The listing builds one solid part. Answer for the finished solid, in the listing's coordinates (mm). Face numbers are marked on the shaded views. A direction names the side the tool comes from. Round coordinates to 2 decimals unless told otherwise and drop trailing zeros. Order: outer loops, then holes, each group sorted by start corner. A loop starts at its lowest first (then second) coordinate and runs counter-clockwise, first axis right, second up. Notation, with made-up numbers: M 63.25,15.5 L 85.25,15.5 A14 ccw 85.25,38.5 Z; hole C 0,59 d4. An arc over 180 degrees is marked long. Put each result on its own line as item: value. Start each with the question number.
1. The mould has two halves that part along X. Classify the marked faces 4 and 5: +X half, -X half, draft (parallel to the pull), parting line (faces both ways), or undercut.
2. The part is cut by section C-C (y = 31.25). Give the vertices of the cut face in (x, z).
3. Which of the six approach directions +Z, -Z, +X, -X, +Y, -Y give full straight-line access (tool end or side, diameter ignored) to the marked faces 1, 2 and 3?
4. The part is cut by section D-D (z = -28.5). Give the vertices of the cut face in (x, y).
5. Each of these flat-tipped pins is pushed along its axis until it touches: pin 1 Ø6 at (x, z) = (58, -15) entering from +Y; pin 2 Ø7 at (x, z) = (15, -16) entering from -Y; pin 3 Ø2 at (y, z) = (30.5, -10.5) entering from -X; pin 4 Ø6.5 at (x, z) = (60, -16) entering from -Y. Where does it stop, or does it pass through?
6. The part is cut by section A-A (y = 23.75). Give the vertices of the cut face in (x, z).
7. Consider line 1 (X direction, y = 32.5, z = -16); line 2 (Z direction, x = 60, y = 25.75); line 3 (X direction, y = 23.75, z = -16). Determine where each line is inside the solid, lowest interval first.
8. The part is cut by section B-B (x = -60). Give the vertices of the cut face in (y, z).
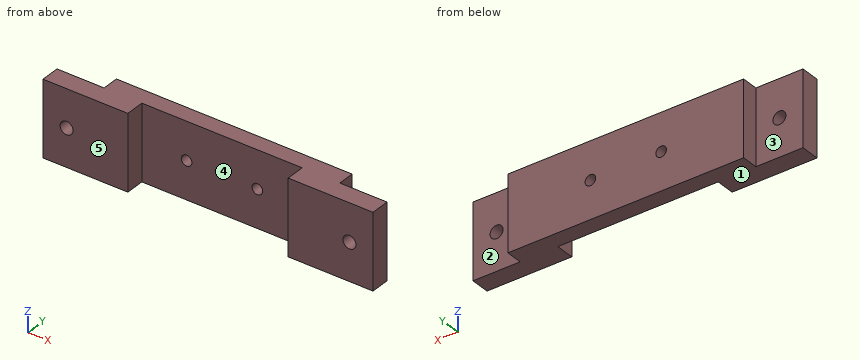
from build123d import *

# Parameters (mm, degrees)
AUFSATZ_LINEAR_AUSTRAGEN1_DEPTH  = 32
F_4_5_4_5_DURCHMESSER_BOHRUNG1_D = 4.5
F_5_5_5_5_DURCHMESSER_BOHRUNG1_D = 5.5


with BuildPart() as part:
    # Skizze1 → Aufsatz-Linear austragen1 (new body)
    with BuildSketch(Plane.XY):
        Polygon((-70, 20), (-34, 20), (-34, 28), (34, 28), (34, 20), (70, 20), (70, 28), (50, 28), (50, 35), (-50, 35), (-50, 28), (-70, 28), align=None)
    extrude(amount=-AUFSATZ_LINEAR_AUSTRAGEN1_DEPTH)

    # Ø4.5 (4.5) Durchmesser Bohrung1 (through all)
    with Locations(Plane(origin=(-15, 28, -16), x_dir=(0, 0, -1), z_dir=(0, -1, 0))):
        with Locations((0, 0), (0, 30)):
            Hole(F_4_5_4_5_DURCHMESSER_BOHRUNG1_D / 2)

    # Ø5.5 (5.5) Durchmesser Bohrung1 (through all)
    with Locations(Plane(origin=(-60, 28, -16), x_dir=(1, 0, 0), z_dir=(0, 1, 0))):
        with Locations((0, 0), (120, 0)):
            Hole(F_5_5_5_5_DURCHMESSER_BOHRUNG1_D / 2)


solid = part.part
Resolved:
1. face 4: undercut
1. face 5: draft
2. outline: M -50,-32 L 50,-32 L 50,0 L -50,0 Z; hole C -15,-16 d4.5; hole C 15,-16 d4.5
3. face 1: -Z, +X, -X, +Y, -Y
3. face 2: +Z, -Z, +X, +Y
3. face 3: +Z, -Z, -X, +Y
4. outline: M -70,20 L -34,20 L -34,28 L 34,28 L 34,20 L 70,20 L 70,28 L 50,28 L 50,35 L -50,35 L -50,28 L -70,28 Z
5. pin 1: y = 28
5. pin 2: y = 28
5. pin 3: x = -50
5. pin 4: y = 20
6. outline: M -70,-32 L -34,-32 L -34,0 L -70,0 Z; M 34,-32 L 70,-32 L 70,0 L 34,0 Z; hole C -60,-16 d5.5; hole C 60,-16 d5.5
7. line 1: -50 to -17.25, -12.75 to 12.75, 17.25 to 50
7. line 2: -32 to -18.75, -13.25 to 0
7. line 3: -70 to -62.75, -57.25 to -34, 34 to 57.25, 62.75 to 70
8. outline: M 20,-32 L 28,-32 L 28,-18.75 L 20,-18.75 Z; M 20,-13.25 L 28,-13.25 L 28,0 L 20,0 Z
